Check sheet for the modelled part. Datum: model origin and axes. Units: mm. Face numbers are marked on the shaded views. A direction names the side the tool comes from. Give positions to 0.01 mm unless a question says otherwise; leave off trailing zeros. Loops run counter-clockwise (first coordinate to the right, second up) from the corner with the lowest first, then second, coordinate; pieces in that order, holes last. Notation, with made-up numbers: (66, 8.5) -> (95, 8.5) arc R24 ccw to (95, 43.5) -> close; hole circle Ø10 at (11.25, 86.5). An arc over 180 degrees is marked (long way). Answer as CSV lines item,"result". Start each with the question number.
(1) Section check D-D on z = 3.5. Enter the section's corners in (x, y), plus the area to 3 significant figures.
(2) Section check C-C on x = 3.5. Enter the section's corners in (y, z), plus the area to 3 significant figures.
(3) Material ranges on line 1 (X direction, y = -18.5, z = 0.25); line 2 (Z direction, x = 3.5, y = -14.25); line 3 (Y direction, x = -20.5, z = 9.25), recorded low to high. Write a range as from..to.
(4) Release check for a two-part mould opening along Y. For the marked faces 1, 2 and 3 record: pulls with the +Y half, pulls with the -Y half, needs draft (parallel to the pull), parting line crosses it, or undercut.
(5) Access from +Z, -Z, +X, -X, +Y, -Y to the whole of each face (thin tool, end or side, straight path). Record for the marked faces 4, 5 and 6.
(6) Section check B-B on y = -16. Enter the section's corners in (x, z), plus the area to 3 significant figures.
(7) Gauge pin test, flat ends, axial feed: pin 1 Ø1.3 at (x, z) = (-21.5, -6) entering from -Y; pin 2 Ø3 at (x, y) = (-14.5, -19.5) entering from -Z; pin 3 Ø1.3 at (x, y) = (-21.5, -20.5) entering from +Z. Record the tip position at first contact, or that the pin passes through.
(8) Section check A-A on z = 1. Enter the section's corners in (x, y), plus the area to 3 significant figures.
from build123d import *

# Parameters (mm, degrees)
BOX009_W           = 32
BOX009_H           = 13
BOX009_DEPTH       = 22
SKETCH066_R        = 12
SKETCH066_R_2      = 1.3
POCKET042006_DEPTH = 8
SKETCH067_R        = 2.15
POCKET042007_DEPTH = 8
SKETCH068_R        = 1.6
POCKET042008_DEPTH = 13.001
SKETCH069_R        = 10.5
POCKET042009_DEPTH = 13.001


with BuildPart() as part:
    # Box009 → Box009 (new body)
    with BuildSketch(Plane(origin=(-24.5, -25, -11), x_dir=(1, 0, 0), z_dir=(0, 0, 1))):
        with Locations((16, 6.5)):
            Rectangle(BOX009_W, BOX009_H)
    extrude(amount=BOX009_DEPTH)

    # Sketch066 (on Face3 of Box009) → Pocket042006 (cut)
    with BuildSketch(Plane(origin=(-24.5, -25, -11), x_dir=(1, 0, 0), z_dir=(0, -1, 0))):
        with Locations((15.576077, -7.031956)):
            Circle(SKETCH066_R)
        with Locations((3.49904, 4.966864)):
            Circle(SKETCH066_R_2)
        with Locations((27.478965, 5.011155)):
            Circle(SKETCH066_R_2)
    extrude(amount=-POCKET042006_DEPTH, mode=Mode.SUBTRACT)

    # Sketch067 (on Face3 of Pocket042006) → Pocket042007 (cut)
    with BuildSketch(Plane(origin=(-24.5, -25, 11), x_dir=(1, 0, 0), z_dir=(0, 0, 1))):
        with Locations((4, 4)):
            Circle(SKETCH067_R)
        with Locations((28, 4)):
            Circle(SKETCH067_R)
    extrude(amount=-POCKET042007_DEPTH, mode=Mode.SUBTRACT)

    # Sketch068 (on Face2 of Pocket042007) → Pocket042008 (cut, through all)
    with BuildSketch(Plane(origin=(-24.5, -25, -11), x_dir=(1, 0, 0), z_dir=(0, -1, 0))):
        with Locations((4, 12)):
            Circle(SKETCH068_R)
        with Locations((28, 12)):
            Circle(SKETCH068_R)
    extrude(amount=-POCKET042008_DEPTH, mode=Mode.SUBTRACT)

    # Sketch069 (on Face2 of Pocket042008) → Pocket042009 (cut, through all)
    with BuildSketch(Plane(origin=(-24.5, -25, -11), x_dir=(1, 0, 0), z_dir=(0, -1, 0))):
        with Locations((38.988731, -2.097178)):
            Circle(SKETCH069_R)
    extrude(amount=-POCKET042009_DEPTH, mode=Mode.SUBTRACT)


solid = part.part
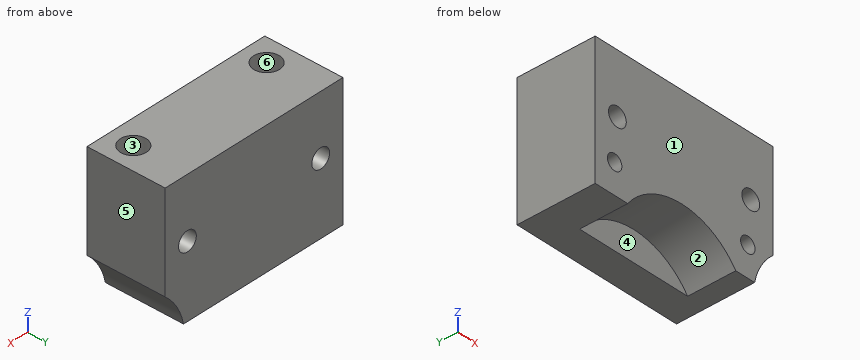
Working result:
1,outline,"(-24.5, -25) -> (7.5, -25) -> (7.5, -12) -> (-24.5, -12) -> close; hole circle Ø4.3 at (-20.5, -21); hole circle Ø4.3 at (3.5, -21)"
1,area,"387 mm^2"
2,outline,"(-25, -11) -> (-12, -11) -> (-12, -0.6) -> (-25, -0.6) -> (-25, -4.8) -> (-17, -4.8) -> (-17, -7.18) -> (-25, -7.18) -> close; (-25, 2.6) -> (-12, 2.6) -> (-12, 11) -> (-18.85, 11) -> (-18.85, 3) -> (-23.15, 3) -> (-23.15, 11) -> (-25, 11) -> close"
2,area,"191 mm^2"
3,line 1,"x = -24.5..-21.91, -19.09..2.09, 4.91..7.5"
3,line 2,"z = -11..-0.6, 2.6..11"
3,line 3,"y = -25..-23.15, -18.85..-12"
4,face 1,"pulls with the -Y half"
4,face 2,"needs draft"
4,face 3,"undercut"
5,face 4,"-Z, -Y"
5,face 5,"+Z, -Z, +X, +Y, -Y"
5,face 6,"+Z"
6,outline,"(-24.5, -11) -> (4.2, -11) arc R10.5 cw to (7.5, -5.26) -> (7.5, 11) -> (-24.5, 11) -> close; hole circle Ø3.2 at (-20.5, 1); hole circle Ø3.2 at (3.5, 1)"
6,area,"676 mm^2"
7,pin 1,"stops at y = -17"
7,pin 2,"stops at z = -8.34"
7,pin 3,"stops at z = 3"
8,outline,"(-24.5, -25) -> (-22.1, -25) -> (-22.1, -12) -> (-24.5, -12) -> close; (-18.9, -25) -> (1.9, -25) -> (1.9, -12) -> (-18.9, -12) -> close; (5.1, -25) -> (7.5, -25) -> (7.5, -12) -> (5.1, -12) -> close"
8,area,"333 mm^2"
